from build123d import *

# Parameters (mm, degrees)
SKETCH2_W           = 0.4
SKETCH2_H           = 2.939387692
CUT_EXTRUDE1_DEPTH  = 10.618211892
SKETCH3_W           = 0.5
SKETCH3_H           = 15
SKETCH3_H_2         = 13
BOSS_EXTRUDE1_DEPTH = 0.125


with BuildPart() as part:
    # Sketch1 → Revolve1 (revolve)
    with BuildSketch(Plane(origin=(0, 0, 0), x_dir=(0, 0, -1), z_dir=(1, 0, 0))):
        with BuildLine():
            Line((0, 0), (2.9, 0))
            Line((2.9, 0), (2.9, 1))
            Line((2.9, 1), (2.5, 1))
            Line((2.5, 1), (2.5, 6.2))
            ThreePointArc((2.5, 6.2), (1.767766953, 7.967766953), (0, 8.7))
            Line((0, 8.7), (0, 0))
        make_face()
    revolve(axis=Axis((0, 0, 0), (0, 1, 0)))

    # Sketch2 → Cut-Extrude1 (cut, through all)
    with BuildSketch(Plane(origin=(0, 0, 0), x_dir=(1, 0, 0), z_dir=(0, 1, 0))):
        with Locations((2.7, 0)):
            Rectangle(SKETCH2_W, SKETCH2_H)
    extrude(amount=CUT_EXTRUDE1_DEPTH, mode=Mode.SUBTRACT)

    # Sketch3 → Boss-Extrude1 (add, symmetric)
    with BuildSketch(Plane.XY):
        with Locations((0.625, -7.5)):
            Rectangle(SKETCH3_W, SKETCH3_H)
        with Locations((1.875, -7.5)):
            Rectangle(SKETCH3_W, SKETCH3_H)
        with Locations((-0.5, -6.5)):
            Rectangle(SKETCH3_W, SKETCH3_H_2)
        with Locations((-1.5, -6.5)):
            Rectangle(SKETCH3_W, SKETCH3_H_2)
    extrude(amount=BOSS_EXTRUDE1_DEPTH, both=True)


solid = part.part
Design review of the part built by this model. Coordinates are the model's own, in mm. A direction names the side the tool comes from. Round coordinates to 2 decimals unless told otherwise and drop trailing zeros. Order: outer loops, then holes, each group sorted by start corner. A loop starts at its lowest first (then second) coordinate and runs counter-clockwise, first axis right, second up. Notation, with made-up numbers: M 36.5,23 L 63.5,23 A21 cw 63.5,62 Z; hole C 89,72 d11. An arc over 180 degrees is marked long. Answer as CSV lines item,"result". Start each with the question number.
1) Add section A-A (y = -11.5). Give the boundary of the cut face in (x, z) (3 decimals), then the cut area to 3 significant figures.
2) Add section B-B (x = 0). Give the boundary of the cut face in (y, z).
3) Add section C-C (z = -1.9). Give the boundary of the cut face in (x, y), then the cut area to 3 significant figures.
4) For pin 1 Ø3 at (y, z) = (-4.5, 0) entering from -X; pin 2 Ø1.5 at (y, z) = (-10.5, -1) entering from -X; pin 3 Ø2 at (y, z) = (-10, -1) entering from +X (3 decimals); pin 4 Ø1.6 at (x, z) = (0.5, 1) entering from +Y, all flat-tipped, find the tip position at first contact; note any pin that passes through.
5) Wall thickness on line 1 along Z through (x, y) = (-1.6, -3) (3 decimals); line 2 along Y through (x, z) = (-2.5, -1.1); line 3 along Y through (x, z) = (0.35, -0.4): over which ranges is each line inside the solid? List them lowest first. Write a range as [from, to].
6) Tool access review of faces 1 (the face through (2.44, 3.64, 0.54)), 2 (the face through (-2.9, 0.5, -0.1)): name each direction out of +Z, -Z, +X, -X, +Y, -Y from which nothing blocks a thin tool from reaching the whole face with its end or side.
7) Add section D-D (x = -1.05). Give the boundary of the cut face in (y, z), then the cut area to 3 significant figures.
Resolved:
1,outline,"M -1.75,-0.125 L -1.25,-0.125 L -1.25,0.125 L -1.75,0.125 Z; M -0.75,-0.125 L -0.25,-0.125 L -0.25,0.125 L -0.75,0.125 Z; M 0.375,-0.125 L 0.875,-0.125 L 0.875,0.125 L 0.375,0.125 Z; M 1.625,-0.125 L 2.125,-0.125 L 2.125,0.125 L 1.625,0.125 Z"
1,area,"0.500 mm^2"
2,outline,"M 0,-2.9 L 1,-2.9 L 1,-2.5 L 6.2,-2.5 A2.5 ccw 6.2,2.5 L 1,2.5 L 1,2.9 L 0,2.9 Z"
3,outline,"M -2.19,0 L 2.19,0 L 2.19,1 L 1.62,1 L 1.62,6.2 A1.62 ccw -1.62,6.2 L -1.62,1 L -2.19,1 Z"
3,area,"25.4 mm^2"
4,pin 1,"x = -1.75"
4,pin 2,"through"
4,pin 3,"x = 2.125"
4,pin 4,"y = 8.68"
5,line 1,"[-0.125, 0.125]"
5,line 2,"[0, 1]"
5,line 3,"[0, 8.64]"
6,face 1,"+Y"
6,face 2,"+Y, -Y"
7,outline,"M 0,-2.7 L 1,-2.7 L 1,-2.27 L 6.2,-2.27 A2.27 ccw 6.2,2.27 L 1,2.27 L 1,2.7 L 0,2.7 Z"
7,area,"37.1 mm^2"
